Input: part model. Units: mm. Frame: model coordinates. A direction names the side the tool comes from. Round coordinates to 2 decimals unless told otherwise and drop trailing zeros. Loops run counter-clockwise (first coordinate to the right, second up) from the corner with the lowest first, then second, coordinate; pieces in that order, holes last. Notation, with made-up numbers: (-5, 57.5) -> (38, 57.5) arc R32 ccw to (38, 83.5) -> close; hole circle Ø11 at (-31, 75.25). An arc over 180 degrees is marked (long way). Answer as a JSON object with one key per item and string values.
```python
from build123d import *

# Parameters (mm, degrees)
RESSALTO_EXTRUS_O1_DEPTH = 2


with BuildPart() as part:
    # Esboço1 → Ressalto-extrusão1 (new body)
    with BuildSketch(Plane(origin=(0, 0, 0), x_dir=(0, 0, -1), z_dir=(1, 0, 0))):
        with BuildLine():
            Line((0, -1.135256663), (0, -19.198580097))
            ThreePointArc((0, -19.198580097), (0.165672539, -19.99560128), (0.635242767, -20.66057794))
            ThreePointArc((0.635242767, -20.66057794), (5.79673997, -22.923055217), (11.239007951, -21.459642756))
            ThreePointArc((11.239007951, -21.459642756), (11.802930255, -20.872546688), (12.086175338, -20.109354458))
            Line((12.086175338, -20.109354458), (13, -14.080459117))
            ThreePointArc((13, -14.080459117), (27.8629628, -1.328429998), (42.670766881, -14.144468704))
            ThreePointArc((42.670766881, -14.144468704), (43.465031593, -15.464843047), (44.962324336, -15.8286552))
            Line((44.962324336, -15.8286552), (54.31286893, -14.347674427))
            ThreePointArc((54.31286893, -14.347674427), (55.520811931, -13.671193843), (56, -12.372297746))
            Line((56, -12.372297746), (56, -0.68631259))
            ThreePointArc((56, -0.68631259), (55.559508665, 0.565858613), (54.432067277, 1.266459252))
            Line((54.432067277, 1.266459252), (42.829728449, 3.833574795))
            ThreePointArc((42.829728449, 3.833574795), (21.542961045, 6.988627316), (0.995627431, 0.594262271))
            ThreePointArc((0.995627431, 0.594262271), (0.2666874, -0.137445342), (0, -1.135256663))
        make_face()
        with BuildLine():
            Line((9, -4.191253682), (9, -15.191253682))
            ThreePointArc((9, -15.191253682), (7, -17.191253682), (5, -15.191253682))
            Line((5, -15.191253682), (5, -4.191253682))
            ThreePointArc((5, -4.191253682), (7, -2.191253682), (9, -4.191253682))
        make_face(mode=Mode.SUBTRACT)
        with BuildLine():
            Line((50, -2.828963065), (50, -9.828963065))
            ThreePointArc((50, -9.828963065), (48, -11.828963065), (46, -9.828963065))
            Line((46, -9.828963065), (46, -2.828963065))
            ThreePointArc((46, -2.828963065), (48, -0.828963065), (50, -2.828963065))
        make_face(mode=Mode.SUBTRACT)
    extrude(amount=RESSALTO_EXTRUS_O1_DEPTH)


solid = part.part
```
1) Section B-B, the plane z = -7. Output: boundary loops of the cut face in (x, y), plus the area to 3 significant figures.
Output:
{"outline": "(0, -22.93) -> (2, -22.93) -> (2, -17.19) -> (0, -17.19) -> close; (0, -2.19) -> (2, -2.19) -> (2, 3.55) -> (0, 3.55) -> close", "area": "22.9 mm^2"}
2) Section D-D, the plane z = -48. Output: boundary loops of the cut face in (x, y), plus the area to 3 significant figures.
Output:
{"outline": "(0, -15.35) -> (2, -15.35) -> (2, -11.83) -> (0, -11.83) -> close; (0, -0.83) -> (2, -0.83) -> (2, 2.69) -> (0, 2.69) -> close", "area": "14.1 mm^2"}
3) Section A-A, the plane x = 0.7. Output: boundary loops of the cut face in (y, z), plus the area to 3 significant figures.
Output:
{"outline": "(-21.46, -11.24) arc R2 ccw to (-20.11, -12.09) -> (-14.08, -13) arc R15 cw to (-14.14, -42.67) arc R2 ccw to (-15.83, -44.96) -> (-14.35, -54.31) arc R2 ccw to (-12.37, -56) -> (-0.69, -56) arc R2 ccw to (1.27, -54.43) -> (3.83, -42.83) arc R48.35 ccw to (0.59, -1) arc R2 ccw to (-1.14, 0) -> (-19.2, 0) arc R2 ccw to (-20.66, -0.64) arc R8.5 ccw to start; hole (-15.19, -9) -> (-4.19, -9) arc R2 ccw to (-4.19, -5) -> (-15.19, -5) arc R2 ccw to start; hole (-9.83, -50) -> (-2.83, -50) arc R2 ccw to (-2.83, -46) -> (-9.83, -46) arc R2 ccw to start", "area": "776 mm^2"}
4) Ray query, probe 1 along Z at (x, y) = (0.2, -9); probe 2 along Z at (x, y) = (0.7, -12); probe 3 along Z at (x, y) = (0.35, -10). Return the intervals inside material, ascending.
Output:
{"probe 1": "z = -56 to -50, -46 to -40.92, -14.74 to -9, -5 to 0", "probe 2": "z = -56 to -42.19, -13.47 to -9, -5 to 0", "probe 3": "z = -56 to -49.99, -46.01 to -41.43, -14.23 to -9, -5 to 0"}
5) Draft query along Z for faces 4 (the face through (0.99, 0.55, -55.57)), 5 (the face through (1, -10, 0)), 6 (the face through (0.99, -2.19, -6.96)). Return one class per face: +Z half, -Z half, draft (parallel to the pull), parting line (faces both ways), or undercut.
Output:
{"face 4": "-Z half", "face 5": "+Z half", "face 6": "undercut"}
6) Reachability of faces 1 (the face through (0.986, -19.985, -0.161)), 2 (the face through (1, -10, -9)), 3 (the face through (0.986, -17.137, -12.537)) from +Z, -Z, +X, -X, +Y, -Y: full face, straight path, thin tool, end or side. Return the list, or none.
Output:
{"face 1": "+Z, +X, -X, -Y", "face 2": "+X, -X", "face 3": "+X, -X, -Y"}
7) Section C-C, the plane y = -7. Output: boundary loops of the cut face in (x, z), plus the area to 3 significant figures.
Output:
{"outline": "(0, -56) -> (2, -56) -> (2, -50) -> (0, -50) -> close; (0, -46) -> (2, -46) -> (2, -39.58) -> (0, -39.58) -> close; (0, -16.08) -> (2, -16.08) -> (2, -9) -> (0, -9) -> close; (0, -5) -> (2, -5) -> (2, 0) -> (0, 0) -> close", "area": "49.0 mm^2"}
